Geometry check sheet. Reference: drawing and pictorial views, mm from the part's lowest x, y, z. Give positions to 0.01 mm unless a question says otherwise; leave off trailing zeros. Loops run counter-clockwise (first coordinate to the right, second up) from the corner with the lowest first, then second, coordinate; pieces in that order, holes last. Notation, with made-up numbers: (-37.5, -17) -> (-20.5, -17) arc R30 ccw to (-20.5, 22) -> close; hole circle Ø3 at (-12, -2). An arc over 180 degrees is marked (long way). Answer in a Markdown table with one row per item. Add a question column.
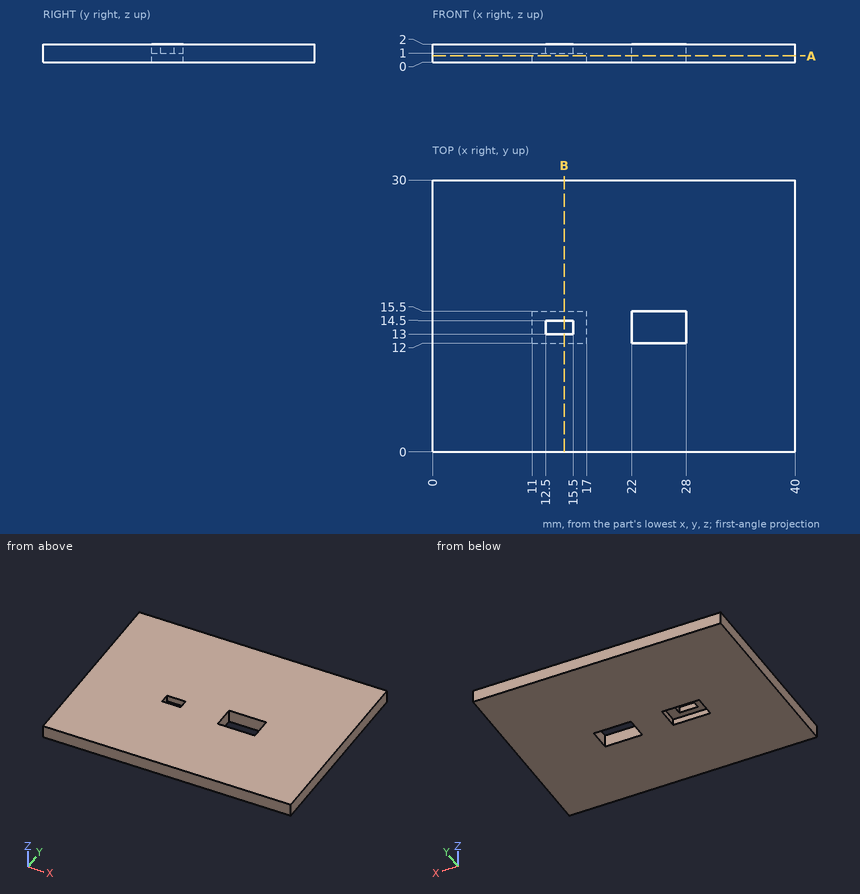
1. Material ranges on L1, parallel to X at y = 14, z = 0.7; L2, parallel to X at y = 13.5, z = 1.7; L3, parallel to Y at x = 23.5, z = 0.6, recorded low to high. Write a range as from..to.
2. Gauge pin test, flat end, axial feed: pin 1 Ø0.5 at (y, z) = (14, 1.5) entering from -X. Record the tip position at first contact, or that the pin passes through.
3. Sectioned sample at A-A (z = 0.7). Enter the section's corners in (x, y).
4. Sectioned sample at B-B (x = 14.5). Enter the section's corners in (y, z), plus the area to 3 significant figures.
Response:
| question | item | result |
|---|---|---|
| 1 | L1 | x = 0..11, 17..22, 28..40 |
| 1 | L2 | x = 0..12.5, 15.5..22, 28..40 |
| 1 | L3 | y = 0..12, 15.5..30 |
| 2 | pin 1 | stops at x = 0 |
| 3 | outline | (0, 0) -> (40, 0) -> (40, 30) -> (0, 30) -> close; hole (11, 12) -> (17, 12) -> (17, 15.5) -> (11, 15.5) -> close; hole (22, 12) -> (28, 12) -> (28, 15.5) -> (22, 15.5) -> close |
| 4 | outline | (0, 0) -> (12, 0) -> (12, 1) -> (13, 1) -> (13, 2) -> (0, 2) -> close; (14.5, 1) -> (15.5, 1) -> (15.5, 0) -> (30, 0) -> (30, 2) -> (14.5, 2) -> close |
| 4 | area | 55.0 mm2 |
